```python
from build123d import *

# Parameters (mm, degrees)
SKETCH025_R     = 22.5
PAD008_DEPTH    = 30
CHAMFER006_SIZE = 2
SKETCH026_W     = 19
SKETCH026_H     = 34.5
POCKET016_DEPTH = 27
POCKET017_DEPTH = 5
SKETCH028_W     = 4
SKETCH028_H     = 4
POCKET018_DEPTH = 23
SKETCH029_W     = 4
SKETCH029_H     = 2
POCKET019_DEPTH = 4
SKETCH030_W     = 4
SKETCH030_H     = 2
POCKET020_DEPTH = 4
SKETCH034_W     = 11
SKETCH034_H     = 34.5
POCKET_DEPTH    = 18
CHAMFER_1_SIZE2 = 3.99
CHAMFER_1_SIZE  = 1.99
CHAMFER_2_SIZE2 = 3.99
CHAMFER_2_SIZE  = 1.99
CHAMFER007_SIZE = 1.99


with BuildPart() as part:
    # Sketch025 → Pad008 (new body)
    with BuildSketch(Plane.XY):
        Circle(SKETCH025_R)
    extrude(amount=PAD008_DEPTH)

    # Chamfer006
    chamfer006_edges = [part.edges().sort_by_distance(p)[0] for p in [
        (-22.5, 0, 0),
    ]]
    chamfer(chamfer006_edges, length=CHAMFER006_SIZE)

    # Sketch026 (on Face3 of Chamfer006) → Pocket016 (cut)
    with BuildSketch(Plane.XY.offset(30)):
        with Locations((0, -0.75)):
            Rectangle(SKETCH026_W, SKETCH026_H)
    extrude(amount=-POCKET016_DEPTH, mode=Mode.SUBTRACT)

    # Sketch027 (on Face6 of Pocket016) → Pocket017 (cut)
    with BuildSketch(Plane(origin=(0, -18, 0), x_dir=(-1, 0, 0), z_dir=(0, 1, 0))):
        with BuildLine():
            ThreePointArc((-3, 9), (-7, 5), (-3, 1))
            Line((-3, 1), (3, 1))
            ThreePointArc((3, 1), (7, 5), (3, 9))
            Line((3, 9), (-3, 9))
        make_face()
    extrude(amount=-POCKET017_DEPTH, mode=Mode.SUBTRACT)

    # Sketch028 (on Face6 of Pocket017) → Pocket018 (cut)
    with BuildSketch(Plane.XY.offset(30)):
        with Locations((-11.5, 12)):
            Rectangle(SKETCH028_W, SKETCH028_H)
        with Locations((-11.5, -7)):
            Rectangle(SKETCH028_W, SKETCH028_H)
        with Locations((11.5, -7)):
            Rectangle(SKETCH028_W, SKETCH028_H)
        with Locations((11.5, 12)):
            Rectangle(SKETCH028_W, SKETCH028_H)
    extrude(amount=-POCKET018_DEPTH, mode=Mode.SUBTRACT)

    # Sketch029 (on Face19 of Pocket018) → Pocket019 (cut)
    with BuildSketch(Plane.YZ.offset(-9.5)):
        with Locations((-11, 27)):
            Rectangle(SKETCH029_W, SKETCH029_H)
        with Locations((8, 27)):
            Rectangle(SKETCH029_W, SKETCH029_H)
        with Locations((8, 8)):
            Rectangle(SKETCH029_W, SKETCH029_H)
    extrude(amount=-POCKET019_DEPTH, mode=Mode.SUBTRACT)

    # Sketch030 (on Face11 of Pocket019) → Pocket020 (cut)
    with BuildSketch(Plane(origin=(9.5, 0, 0), x_dir=(0, -1, 0), z_dir=(-1, 0, 0))):
        with Locations((-8, 8)):
            Rectangle(SKETCH030_W, SKETCH030_H)
        with Locations((-8, 27)):
            Rectangle(SKETCH030_W, SKETCH030_H)
        with Locations((11, 8)):
            Rectangle(SKETCH030_W, SKETCH030_H)
        with Locations((11, 27)):
            Rectangle(SKETCH030_W, SKETCH030_H)
    extrude(amount=-POCKET020_DEPTH, mode=Mode.SUBTRACT)

    # Sketch034 (on Face6 of Pocket020) → Pocket (cut)
    with BuildSketch(Plane.XY.offset(30)):
        with Locations((-5.5, -0.75)):
            Rectangle(SKETCH034_W, SKETCH034_H)
    extrude(amount=-POCKET_DEPTH, mode=Mode.SUBTRACT)

    # Chamfer 1
    chamfer_1_edges = [part.edges().sort_by_distance(p)[0] for p in [
        (9.5, 8, 28),
        (9.5, -11, 28),
        (9.5, -11, 9),
        (9.5, 8, 9),
    ]]
    chamfer_1_side = part.faces().sort_by_distance((9.5, -1.552236, 15.94095))[0]
    chamfer(chamfer_1_edges, length=CHAMFER_1_SIZE, length2=CHAMFER_1_SIZE2, reference=chamfer_1_side)

    # Chamfer 2
    chamfer_2_edges = [part.edges().sort_by_distance(p)[0] for p in [
        (-9.5, 8, 9),
    ]]
    chamfer_2_side = part.faces().sort_by_distance((-9.5, -1.511905, 7.18))[0]
    chamfer(chamfer_2_edges, length=CHAMFER_2_SIZE, length2=CHAMFER_2_SIZE2, reference=chamfer_2_side)

    # Chamfer007
    chamfer007_edges = [part.edges().sort_by_distance(p)[0] for p in [
        (-11, 8, 28),
        (-11, -11, 28),
    ]]
    chamfer(chamfer007_edges, length=CHAMFER007_SIZE)


solid = part.part
```
Geometry: final body of the model. Coordinates: model frame, mm. A direction names the side the tool comes from. Give positions to 0.01 mm unless a question says otherwise; leave off trailing zeros. Write each loop counter-clockwise with the first axis right and the second up, starting at its lowest first coordinate (ties: lowest second). Pieces come first, ordered by that corner, then holes.
1. Section query C-C, the plane y = 0. Return loops of the section in (x, z), then the cut area to 3 significant figures.
2. Draft query along Z for faces 1 (the flat face through (-12, -7, 7)), 2 (the cylindrical face through (7, -20, 5)), 3 (the flat face through (-13, -9, 29)). Return one class per face: released by +Z, released by -Z, zero draft, split by the parting line, or undercut.
3. Line query: probe 1 along X at (y, z) = (0, 28.5); probe 2 along Y at (x, z) = (10.5, 13.5); probe 3 along Z at (x, y) = (-10.5, 5.5). Output: solid intervals per line, ascending.
4. Section query B-B, the plane z = 19.5. Return loops of the section in (x, y).
5. Section query A-A, the plane x = 0. Return loops of the section in (y, z).
6. Pin query (flat end, axial travel): P1, Ø6, axis at y = 13.5, z = 3.5, coming from the -X side; P2, Ø8, axis at x = 5.5, y = 1.5, coming from the -Z side; P3, Ø12, axis at x = -9, z = 15.5, coming from the -Y side; P4, Ø2, axis at x = -11, z = 13, coming from the -Y side. Return the tip coordinate at first contact, or that it passes through.
7. Reachability of faces 4 (the flat face through (11, -9, 18)), 5 (the flat face through (11.523, 8.028, 28.981)) from +Z, -Z, +X, -X, +Y, -Y: full face, straight path, thin tool, end or side. Return the list, or none.
8. Section query D-D, the plane z = 5. Return loops of the section in (x, y), then the cut area to 3 significant figures.
Computed:
1. outline: (-22.5, 2) - (-20.5, 0) - (20.5, 0) - (22.5, 2) - (22.5, 30) - (9.5, 30) - (9.5, 3) - (-9.5, 3) - (-9.5, 12) - (-11, 12) - (-11, 30) - (-22.5, 30) - close
1. area: 806 mm2
2. face 1: released by +Z
2. face 2: undercut
2. face 3: zero draft
3. probe 1: x = -22.5 to -11, 9.5 to 22.5
3. probe 2: y = -19.9 to -9, -5 to 10, 14 to 19.9
3. probe 3: z = 0 to 12
4. outline: circle Ø45 at (0, 0); hole (-13.5, -9) - (-11, -9) - (-11, -18) - (9.5, -18) - (9.5, -9) - (13.5, -9) - (13.5, -5) - (9.5, -5) - (9.5, 10) - (13.5, 10) - (13.5, 14) - (9.5, 14) - (9.5, 16.5) - (-11, 16.5) - (-11, 14) - (-13.5, 14) - (-13.5, 10) - (-11, 10) - (-11, -5) - (-13.5, -5) - close
5. outline: (-22.5, 9) - (-18, 9) - (-18, 30) - (-22.5, 30) - close; (-21.5, 1) - (-20.5, 0) - (20.5, 0) - (22.5, 2) - (22.5, 30) - (16.5, 30) - (16.5, 3) - (-18, 3) - (-18, 1) - close
6. P1: stops at x = -19.9
6. P2: stops at z = 0
6. P3: stops at y = -22.3
6. P4: stops at y = -20.16
7. face 4: +Z
7. face 5: none
8. outline: (-9.5, -18) - (-9.5, 16.5) - (9.5, 16.5) - (9.5, -18) - (7, -18) - (7, -21.38) arc R22.5 ccw (long way) to (-7, -21.38) - (-7, -18) - close
8. area: 877 mm2
